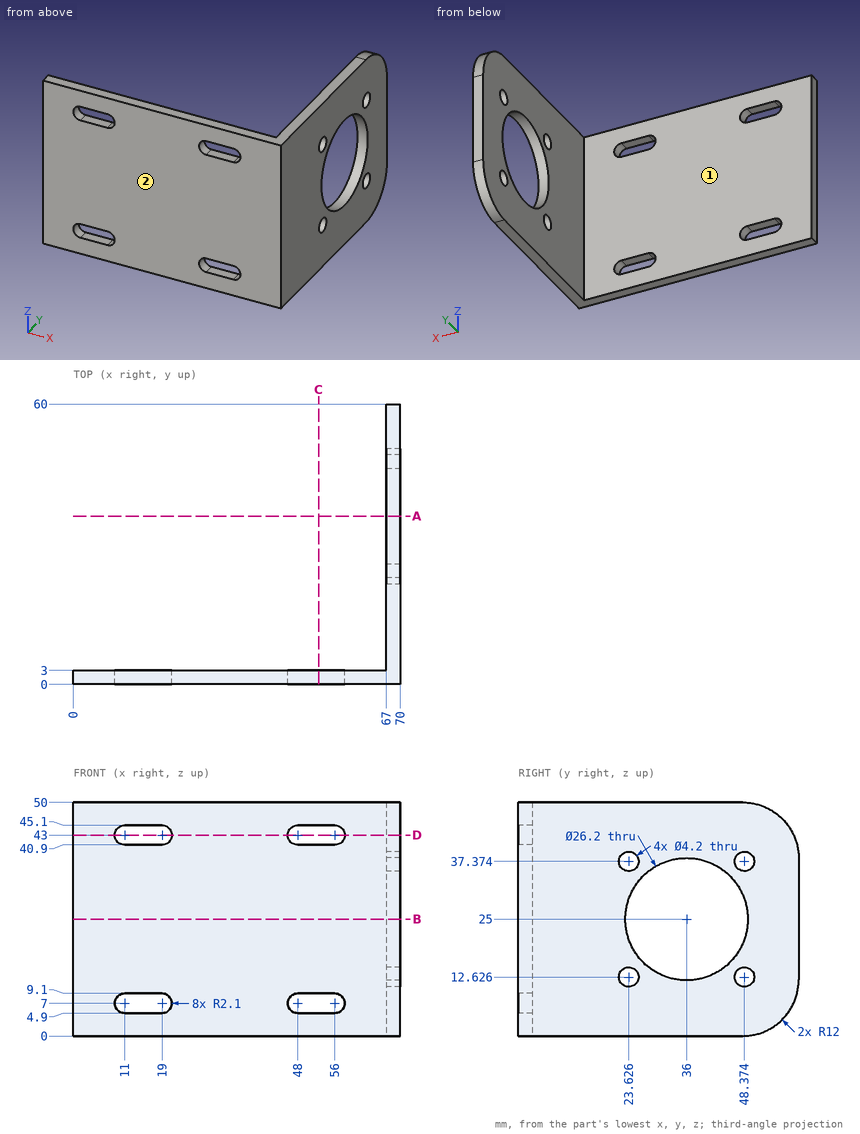
Geometry check sheet. Reference: drawing and pictorial views, mm from the part's lowest x, y, z. A direction names the side the tool comes from. Coordinates: 2 decimals unless noted, no trailing zeros. Write each loop counter-clockwise with the first axis right and the second up, starting at its lowest first coordinate (ties: lowest second). Pieces come first, ordered by that corner, then holes. Notation, with made-up numbers: (37.5, 70.5) - (86.5, 70.5) arc R21 cw to (86.5, 75.5) - close; hole circle Ø4 at (83.5, 35). An arc over 180 degrees is marked (long way). Write item = value, one per line.
Q1. Go/stop test with flat-tipped pins: pin 1 Ø3.5 at (x, y) = (16.5, 1.5) entering from -Z; pin 2 Ø8 at (y, z) = (49.5, 9) entering from -X; pin 3 Ø4 at (y, z) = (23.63, 12.63) entering from -X; pin 4 Ø5 at (x, z) = (10.5, 22) entering from +Y. Record where each tip stops, or that it passes through.
Answer:
pin_1 = 0
pin_2 = 67
pin_3 = through
pin_4 = 3
Q2. Cross-section at B-B (z = 25). Enter the section's corners in (x, y).
Answer:
outline = (0, 0) - (70, 0) - (70, 22.9) - (67, 22.9) - (67, 3) - (0, 3) - close; (67, 49.1) - (70, 49.1) - (70, 60) - (67, 60) - close
Q3. Cross-section at A-A (y = 36). Enter the section's corners in (x, z), plus the area to 3 significant figures.
Answer:
outline = (67, 0) - (70, 0) - (70, 11.9) - (67, 11.9) - close; (67, 38.1) - (70, 38.1) - (70, 50) - (67, 50) - close
area = 71.4 mm²
Q4. Cross-section at C-C (x = 52.5). Enter the section's corners in (y, z).
Answer:
outline = (0, 0) - (3, 0) - (3, 4.9) - (0, 4.9) - close; (0, 9.1) - (3, 9.1) - (3, 40.9) - (0, 40.9) - close; (0, 45.1) - (3, 45.1) - (3, 50) - (0, 50) - close
Q5. Cross-section at D-D (z = 43). Enter the section's corners in (x, y).
Answer:
outline = (0, 0) - (8.9, 0) - (8.9, 3) - (0, 3) - close; (21.1, 0) - (45.9, 0) - (45.9, 3) - (21.1, 3) - close; (58.1, 0) - (70, 0) - (70, 58.91) - (67, 58.91) - (67, 3) - (58.1, 3) - close
Q6. Material ranges on L1, parallel to Y at x = 54, z = 48.5; L2, parallel to Z at x = 69.1, y = 36; L3, parallel to X at y = 30, z = 12, recorded low to high. Write a range as from..to.
Answer:
L1 = 0..3
L2 = 0..11.9, 38.1..50
L3 = 67..70
Q7. Access from +Z, -Z, +X, -X, +Y, -Y to the whole of each face (thin tool, end or side, straight path). Record for the marked faces 1 and 2.
Answer:
face_1 = +Z, -Z, -X, +Y
face_2 = +Z, -Z, +X, -X, -Y
